Read the model definition and answer for the solid it produces. Units are mm, in the model's axes. A direction names the side the tool comes from. Give positions to 0.01 mm unless a question says otherwise; leave off trailing zeros. Write each loop counter-clockwise with the first axis right and the second up, starting at its lowest first coordinate (ties: lowest second). Pieces come first, ordered by that corner, then holes.
```python
from build123d import *
from build123d.topology import SkipClean

# Parameters (mm, degrees)
SKETCH1_R           = 30
SKETCH1_R_2         = 15
BOSS_EXTRUDE1_DEPTH = 30
SKETCH2_R           = 30
SKETCH2_R_2         = 15
BOSS_EXTRUDE2_DEPTH = 32.5
CUT_EXTRUDE2_START  = 32.5
SKETCH2_3_R         = 15
CUT_EXTRUDE2_DEPTH  = 15
BOSS_EXTRUDE3_START = -30
SKETCH1_4_R         = 15
BOSS_EXTRUDE3_DEPTH = 15


with BuildPart() as part:
    # Sketch1 → Boss-Extrude1 (new, symmetric)
    with BuildSketch(Plane.XY):
        Circle(SKETCH1_R)
        Circle(SKETCH1_R_2, mode=Mode.SUBTRACT)
        Circle(SKETCH1_R_2)
    extrude(amount=BOSS_EXTRUDE1_DEPTH, both=True)

    # Sketch2 → Boss-Extrude2 (add)
    with SkipClean():  # the faces are left unmerged after this step: merging them gives an invalid solid
        with BuildSketch(Plane(origin=(0, 0, 0), x_dir=(1, 0, 0), z_dir=(0, 1, 0))):
            with Locations(Location((0, 0, 0), (0, 0, 270))):
                Circle(SKETCH2_R)
            Circle(SKETCH2_R_2, mode=Mode.SUBTRACT)
            Circle(SKETCH2_R_2)
        extrude(amount=BOSS_EXTRUDE2_DEPTH)

    # Sketch2<3> → Cut-Extrude2 (cut)
    with SkipClean():  # the faces are left unmerged after this step: merging them gives an invalid solid
        with BuildSketch(Plane(origin=(0, 0, 0), x_dir=(1, 0, 0), z_dir=(0, 1, 0)).offset(CUT_EXTRUDE2_START)):
            with Locations(Location((0, 0, 0), (0, 0, 270))):
                Circle(SKETCH2_3_R)
        extrude(amount=-CUT_EXTRUDE2_DEPTH, mode=Mode.SUBTRACT)

    # Sketch1<4> → Boss-Extrude3 (add)
    with SkipClean():  # the faces are left unmerged after this step: merging them gives an invalid solid
        with BuildSketch(Plane.XY.offset(BOSS_EXTRUDE3_START)):
            Circle(SKETCH1_4_R)
        extrude(amount=-BOSS_EXTRUDE3_DEPTH)


solid = part.part
```
Item 1: Section A-A (x = 20.5) is taken. Write down the section's boundary in (y, z), and give its area (3 significant figures).
Result set:
outline: (-21.9, -30) - (21.9, -30) - (21.9, -21.9) - (32.5, -21.9) - (32.5, 21.9) - (21.9, 21.9) - (21.9, 30) - (-21.9, 30) - close
area: 3,090 mm2
Item 2: Which of the six approach directions +Z, -Z, +X, -X, +Y, -Y give full straight-line access (tool end or side, diameter ignored) to faces 1 (the cylindrical face through (-14.985, 0.66, -37.395)), 2 (the flat face through (0, 0, 30)), 3 (the cylindrical face through (0.66, 25.105, -14.985))?
Result set:
face 1: -Z
face 2: +Z, +X, -X, +Y, -Y
face 3: +Y
Item 3: Section D-D (x = 5.5) is taken. Write down the section's boundary in (y, z), and give its area (3 significant figures).
Result set:
outline: (-29.49, -30) - (-13.96, -30) - (-13.96, -45) - (13.96, -45) - (13.96, -30) - (29.49, -30) - (29.49, -29.49) - (32.5, -29.49) - (32.5, -13.96) - (17.5, -13.96) - (17.5, 13.96) - (32.5, 13.96) - (32.5, 29.49) - (29.49, 29.49) - (29.49, 30) - (-29.49, 30) - close
area: 3,720 mm2
Item 4: Find the intervals of material crossed by line 1 along X through (y, z) = (23, 0); line 2 along Z through (x, y) = (26.5, -7.5); line 3 along X through (y, z) = (4.5, -37.5), in increasing order.
Result set:
line 1: x = -30 to -15, 15 to 30
line 2: z = -30 to 30
line 3: x = -14.31 to 14.31
Item 5: Each of these flat-tipped pins is pushed along its axis until it touches: pin 1 Ø4 at (x, y) = (18, -19.5) entering from -Z; pin 2 Ø6 at (y, z) = (11, -6) entering from +X; pin 3 Ø1.5 at (y, z) = (-2, -16.5) entering from +X. Where does it stop, or does it pass through?
Result set:
pin 1: stops at z = -30
pin 2: stops at x = 29.85
pin 3: stops at x = 29.97
Item 6: Section B-B (z = 8.5) is taken. Write down the section's boundary in (x, y), and give its area (3 significant figures).
Result set:
outline: (-28.77, 8.5) arc R30 ccw (long way) to (28.77, 8.5) - (28.77, 32.5) - (12.36, 32.5) - (12.36, 17.5) - (-12.36, 17.5) - (-12.36, 32.5) - (-28.77, 32.5) - close
area: 2,930 mm2
Item 7: Section C-C (y = -24) is taken. Write down the section's boundary in (x, z), and give its area (3 significant figures).
Result set:
outline: (-18, -30) - (18, -30) - (18, 30) - (-18, 30) - close
area: 2,160 mm2
